Geometry check sheet. Reference: drawing and pictorial views, mm from the part's lowest x, y, z. A direction names the side the tool comes from. Coordinates: 2 decimals unless noted, no trailing zeros. Loops run counter-clockwise (first coordinate to the right, second up) from the corner with the lowest first, then second, coordinate; pieces in that order, holes last.
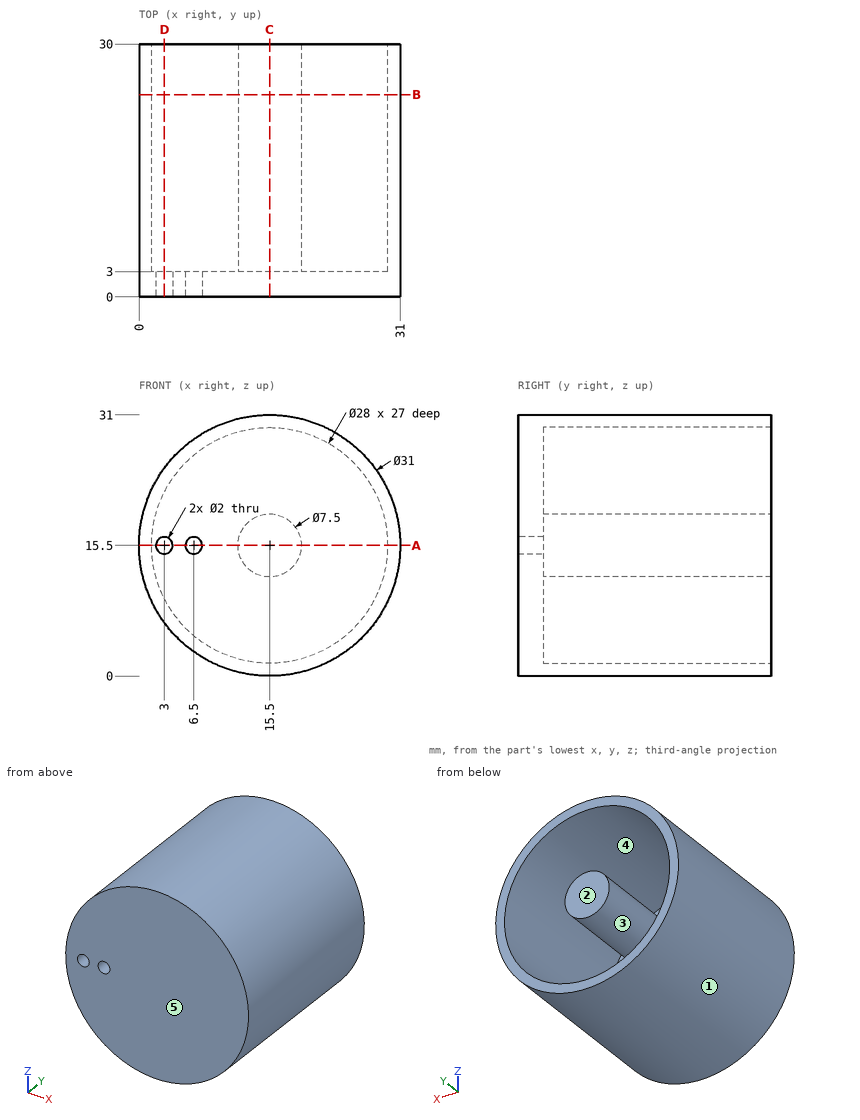
1) Access from +Z, -Z, +X, -X, +Y, -Y to the whole of each face (thin tool, end or side, straight path). Record for the marked faces 4 and 5.
Data:
face 4: +Y
face 5: +Z, -Z, +X, -X, -Y
2) Section check B-B on y = 24. Record the cut outline in (x, z), and give its area (3 significant figures).
Data:
outline: circle Ø31 at (15.5, 15.5); circle Ø7.5 at (15.5, 15.5); hole circle Ø28 at (15.5, 15.5)
area: 183 mm2
3) Mould release check, pull along Z, two halves, no side actions. Record for the marked faces 1, 2 and 3: +Z half, -Z half, draft (parallel to the pull), parting line (faces both ways), or undercut.
Data:
face 1: parting line
face 2: draft
face 3: undercut
4) Section check A-A on z = 15.5. Record the cut outline in (x, y), and give its area (4 significant figures).
Data:
outline: (0, 0) - (2, 0) - (2, 3) - (1.5, 3) - (1.5, 30) - (0, 30) - close; (4, 0) - (5.5, 0) - (5.5, 3) - (4, 3) - close; (7.5, 0) - (31, 0) - (31, 30) - (29.5, 30) - (29.5, 3) - (19.25, 3) - (19.25, 30) - (11.75, 30) - (11.75, 3) - (7.5, 3) - close
area: 364.5 mm2
5) Section check D-D on x = 3. Record the cut outline in (y, z), and give its area (3 significant figures).
Data:
outline: (0, 6.33) - (30, 6.33) - (30, 9.2) - (3, 9.2) - (3, 14.5) - (0, 14.5) - close; (0, 16.5) - (3, 16.5) - (3, 21.8) - (30, 21.8) - (30, 24.67) - (0, 24.67) - close
area: 203 mm2
6) Depth check by flat-ended pin: pin 1 (3 mm diameter, centred on x = 10, y = 22.5, fed in from +Z) (3 decimals); pin 2 (1.5 mm diameter, centred on x = 16.5, y = 26.5, fed in from -Z); pin 3 (1.8 mm diameter, centred on x = 6.5, z = 15.5, fed in from +Y); pin 4 (10 mm diameter, centred on y = 15, z = 3.5, fed in from -X). Enter the tip coordinate at first touch or a pass-through.
Data:
pin 1: stops at z = 30.475
pin 2: stops at z = 0
pin 3: passes through
pin 4: stops at x = 1.67
7) Material ranges on probe 1 along X at (y, z) = (1.65, 15.5); probe 2 along X at (y, z) = (11, 14); probe 3 along Y at (x, z) = (23, 22.5), recorded low to high.
Data:
probe 1: x = 0 to 2, 4 to 5.5, 7.5 to 31
probe 2: x = 0.07 to 1.58, 12.06 to 18.94, 29.42 to 30.93
probe 3: y = 0 to 3
8) Section check C-C on x = 15.5. Record the cut outline in (y, z).
Data:
outline: (0, 0) - (30, 0) - (30, 1.5) - (3, 1.5) - (3, 11.75) - (30, 11.75) - (30, 19.25) - (3, 19.25) - (3, 29.5) - (30, 29.5) - (30, 31) - (0, 31) - close
